The model under review builds one solid part; all positions refer to its coordinate system, in mm. A direction names the side the tool comes from. Coordinates: 2 decimals unless noted, no trailing zeros. Loops run counter-clockwise (first coordinate to the right, second up) from the corner with the lowest first, then second, coordinate; pieces in that order, holes last. Notation, with made-up numbers: (13, 62) - (72, 62) arc R11 ccw to (72, 80) - close; hole circle Ø6 at (43.25, -30). An arc over 180 degrees is marked (long way). Use a Markdown table: item, result. Add a question column.
1) For faces 1 (the flat face through (10, -3, -11)), 2 (the cylindrical face through (12.059, -0.088, -7.102)), 3 (the flat face through (6.55, -1, -7)), 4 (the flat face through (-7.08, 5.17, -0.25)), list the 3-axis set-ups (+Z, -Z, +X, -X, +Y, -Y) from which the entire face can be reached by the end or side of a thin tool; tool diameter is ignored.
2) Clearance check with flat-ended pins moving along their axes: pin 1 (0.5 mm diameter, centred on x = 11, z = -8, fed in from -Y); pin 2 (6.5 mm diameter, centred on y = -1, z = -8.5, fed in from +X); pin 3 (0.7 mm diameter, centred on x = 10, z = -10.5, fed in from -Y). State where each tip first meets the part, or that it passes through.
3) The part is to be moulded in two halves that separate along Y. For faces 5 (the cylindrical face through (-4.336, -19.524, -2.021)), 6 (the cylindrical face through (9.32, -4.22, -8.92)), 7 (the flat face through (-0.936, -8.72, -0.253)), say which applies: pulls with the +Y half, pulls with the -Y half, needs draft (parallel to the pull), parting line crosses it, or undercut.
4) To check wall thickness, follow L1, parallel to X at y = -5, z = -3.5; L2, parallel to Y at x = 9, z = -1.75; L3, parallel to Z at x = -2, y = -18. State the ranges of each line that lie inside material, in increasing order. Write a range as [from, to].
5) Add section A-A, the plane z = -4.75. Give the boundary of the cut face in (x, y).
6) Add section B-B, the plane z = -9.1. Give the boundary of the cut face in (x, y).
Autodesk Fusion 360 part; units mm, degrees
sketch "Esquisse1" plane through (0, 0, 0) normal (0, 0, 1) x (1, 0, 0)
  circle A0 centre (0, 0) radius 20
  line L0 (19.7661, -3.05) -> (8.2661, -3.05)
  line L1 (8.2661, -3.05) -> (8.2661, 3.1)
  line L2 (14.3661, 3.05) -> (19.7661, 3.05)
  line L3 (8.2661, -3.05) -> (14.4602, -3.05)
  line L4 (14.3661, 10.35) -> (8.2661, 10.35)
  line L5 (8.2661, 10.35) -> (8.2661, -3.05)
  line L6 (0, 0) -> (29, 0) construction
  line L7 (14.3661, 3.05) -> (14.3661, 10.35)
  line L8 (-9.8244, 10.9164) -> (-16.1464, 7.2664)
  line L9 (-16.1464, 7.2664) -> (-13.0964, 1.9836)
  line L10 (-13.0964, 1.9836) -> (-1.4917, 8.6836)
  line L11 (-1.4917, 8.6836) -> (-4.5887, 14.0479)
  line L12 (-7.2417, 18.6429) -> (-1.4917, 8.6836)
  line L13 (-9.8244, 10.9164) -> (-12.5244, 15.5929)
  line L14 (-4.5417, -13.9664) -> (1.7803, -17.6164)
  line L15 (1.7803, -17.6164) -> (4.8303, -12.3336)
  line L16 (4.8303, -12.3336) -> (-6.7744, -5.6336)
  line L17 (-6.7744, -5.6336) -> (-9.8715, -10.9979)
  line L18 (-12.5244, -15.5929) -> (-6.7744, -5.6336)
  line L19 (-4.5417, -13.9664) -> (-7.2417, -18.6429)
  circle A1 centre (2.9108, 13.6941) radius 1.75
  line L20 (0, 0) -> (2.9108, 13.6941) construction
  circle A2 centre (-13.3148, -4.3262) radius 1.75
  circle A3 centre (10.404, -9.3678) radius 1.75
  line L21 (6.55, 3.7816) -> (0, 7.5633)
  line L22 (0, 7.5633) -> (-6.55, 3.7816)
  line L23 (-6.55, 3.7816) -> (-6.55, -3.7816)
  line L24 (-6.55, -3.7816) -> (0, -7.5633)
  line L25 (0, -7.5633) -> (6.55, -3.7816)
  line L26 (6.55, -3.7816) -> (6.55, 3.7816)
  dimension "d1" = 40
  dimension "d2" = 6.1
  dimension "d3" = 11.5
  dimension "d6" = 6.1
  dimension "d7" = 3.05
  dimension "d8" = 13.4
  dimension "d10" = 360
  dimension "d16" = 3.5
  dimension "d17" = 78
  dimension "d19" = 360
  dimension "d21" = 14
  dimension "d25" = 6.55
extrude "Extrusion1" add sketch "Esquisse1" against normal blind 4.1 contours A0 L0 L1 L2 L3 L4 L5 L7 | A0 L0 L1 L2 L3 L4 L5 L7 L8 L9 L10 L11 L12 L13 L14 L15 L16 L17 L18 L19 | A0 L8 L9 L10 L11 L12 L13 | A0 L14 L15 L16 L17 L18 L19 | A1 | A2 | A3 | L21 L22 L23 L24 L25 L26
extrude "Extrusion2" cut sketch "Esquisse1" against normal blind 2.1 contours A0 L0 L1 L2 L3 L4 L5 L7 | A0 L8 L9 L10 L11 L12 L13 | A0 L14 L15 L16 L17 L18 L19
chamfer "Chanfrein1" distance 0.5 angle 45 15 edges at (-4.3667, 13.6633, 0) (-11.1744, 13.2546, 0) (-12.9854, 9.0914, 0) (-14.6214, 4.625, 0) (-7.294, 5.3336, 0) (-9.6494, -10.6133, 0) (-0.972, -8.9836, 0) (-5.8917, -16.3046, 0) (-1.3807, -15.7914, 0) (3.3053, -14.975, 0) (8.2661, 3.65, 0) (14.0161, -3.05, 0) (17.0661, 3.05, 0) (14.3661, 6.7, 0) (11.3161, 10.35, 0)
extrude "Extrusion5" cut sketch "Esquisse1" against normal blind 4.1 contours A1 | A2 | A3
extrude "Extrusion6" cut sketch "Esquisse1" against normal blind 4.1 contours L21 L22 L23 L24 L25 L26
chamfer "Chanfrein4" distance 0.5 angle 45 6 edges at (-6.55, 0, 0) (-3.275, 5.6725, 0) (3.275, 5.6725, 0) (6.55, 0, 0) (3.275, -5.6725, 0) (-3.275, -5.6725, 0)
sketch "Esquisse2" plane through (0, 0, -4.1) normal (0, 0, -1) x (1, 0, 0)
  circle A0 centre (0, 0) radius 20
  circle A1 centre (2.9108, -13.6941) radius 1.75
  circle A2 centre (10.404, 9.3678) radius 1.75
  circle A3 centre (-13.3148, 4.3262) radius 1.75
  line L0 (9.1652, 4) -> (13.2, 4)
  line L1 (13.2, 4) -> (13.2, -4)
  line L2 (13.2, -4) -> (9.1652, -4)
  arc A4 (9.1652, 4) -> (9.1652, -4) centre (0, 0) ccw
  line L3 (6.55, -3.7816) -> (0, -7.5633)
  line L4 (0, -7.5633) -> (-6.55, -3.7816)
  line L5 (-6.55, -3.7816) -> (-6.55, 3.7816)
  line L6 (-6.55, 3.7816) -> (0, 7.5633)
  line L7 (0, 7.5633) -> (6.55, 3.7816)
  line L8 (6.55, 3.7816) -> (6.55, -3.7816)
  dimension "d36" = 20
  dimension "d37" = 8
  dimension "d39" = 4
extrude "Extrusion7" add sketch "Esquisse2" along normal blind 10 contours L0 L1 L2 A4
ref_plane "Plan de construction2" through (8.55, 0, -7.3) normal (-1, 0, 0) x (0, 1, 0)
sketch "Esquisse3" plane through (8.55, 0, 0) normal (-1, 0, 0) x (0, 1, 0)
  line L0 (4, -4.1) -> (-4, -4.1)
  line L1 (-4, -4.1) -> (-4, -14.1)
  line L2 (-4, -14.1) -> (4, -14.1)
  line L3 (4, -14.1) -> (4, -4.1)
  line L4 (-3, -14.1) -> (3, -14.1)
  line L5 (3, -14.1) -> (3, -9.1)
  line L6 (3, -9.1) -> (-3, -9.1) construction
  line L7 (-3, -9.1) -> (-3, -14.1)
  line L8 (3, -7.3679) -> (0, -5.6359)
  line L9 (0, -5.6359) -> (-3, -7.3679)
  line L10 (-3, -7.3679) -> (-3, -10.8321)
  line L11 (3, -10.8321) -> (3, -7.3679)
  line L12 (10.85, 0) -> (-3.55, 0)
  line L13 (3, 9.1) -> (-3, 9.1) construction
  line L14 (0, 5.6359) -> (-3, 7.3679)
  line L15 (3, 10.8321) -> (3, 7.3679)
  line L16 (-4, 14.1) -> (4, 14.1)
  line L17 (4, 4.1) -> (-4, 4.1)
  line L18 (-3, 14.1) -> (3, 14.1)
  line L19 (-3, 9.1) -> (-3, 14.1)
  line L20 (3, 14.1) -> (3, 9.1)
  line L21 (3, 7.3679) -> (0, 5.6359)
  line L22 (-4, 4.1) -> (-4, 14.1)
  line L23 (-3, 7.3679) -> (-3, 10.8321)
  line L24 (4, 14.1) -> (4, 4.1)
  point P0 (0, -9.1)
  point P1 (0, 9.1)
  dimension "d42" = 5
  dimension "d43" = 6
  dimension "d44" = 1
extrude "Extrusion8" cut sketch "Esquisse3" against normal blind 2.4 contours L14 L15 L16 L18 L19 L20 L21 L23
hole "Perçage1" at (13.2, 0, -9.1) direction (-1, 0, 0) diameter 4 depth 7 tip angle 180
fillet "Congé1" radius 1.5 4 edges at (13.2, -4, -9.1) (13.2, 4, -9.1) (9.1652, 4, -9.1) (9.1652, -4, -9.1)
fillet "Congé2" radius 0.5 8 edges at (10.8998, -4, -14.1) (9.3334, -4.2104, -14.1) (-10, 0, -14.1) (9.3334, 4.2104, -14.1) (10.8998, 4, -14.1) (12.7607, 3.5607, -14.1) (13.2, 0, -14.1) (12.7607, -3.5607, -14.1)
equation "d6 = d2"
equation "d7 = d2 / 2"
equation "d39 = d37 / 2"
equation "d44 = ( 8 mm - d43 ) / 2"
From the geometry:
| question | item | result |
|---|---|---|
| 1 | face 1 | -Z |
| 1 | face 2 | +X |
| 1 | face 3 | +Z, -Z |
| 1 | face 4 | +Z |
| 2 | pin 1 | stops at y = -4 |
| 2 | pin 2 | stops at x = 13.2 |
| 2 | pin 3 | stops at y = -4.07 |
| 3 | face 5 | parting line crosses it |
| 3 | face 6 | pulls with the -Y half |
| 3 | face 7 | undercut |
| 4 | L1 | x = [-19.36, -14.93], [-11.7, -4.44], [4.44, 19.36] |
| 4 | L2 | y = [-17.86, -10.41], [-8.32, -3.05], [10.35, 17.86] |
| 4 | L3 | z = [-4.1, 0] |
| 5 | outline | (8.78, -4.78) arc R1.5 cw to (10.1, -4) - (11.7, -4) arc R1.5 ccw to (13.2, -2.5) - (13.2, 2.5) arc R1.5 ccw to (11.7, 4) - (10.1, 4) arc R1.5 cw to (8.78, 4.78) arc R10 ccw (long way) to start; hole (-6.55, -3.78) - (0, -7.56) - (6.55, -3.78) - (6.55, 3.78) - (0, 7.56) - (-6.55, 3.78) - close |
| 6 | outline | (-6.55, -3.78) - (-6.55, 3.78) - (0, 7.56) - (6.55, 3.78) - (6.55, 2) - (8.55, 2) - (8.55, 3) - (10.95, 3) - (10.95, 2) - (13.2, 2) - (13.2, 2.5) arc R1.5 ccw to (11.7, 4) - (10.1, 4) arc R1.5 cw to (8.78, 4.78) arc R10 ccw (long way) to (8.78, -4.78) arc R1.5 cw to (10.1, -4) - (11.7, -4) arc R1.5 ccw to (13.2, -2.5) - (13.2, -2) - (10.95, -2) - (10.95, -3) - (8.55, -3) - (8.55, -2) - (6.55, -2) - (6.55, -3.78) - (0, -7.56) - close |
